```python
from build123d import *

# Parameters (mm, degrees)
BOSS_EXTRUDE1_DEPTH = 1.524
SKETCH2_R           = 7.874
BOSS_EXTRUDE2_DEPTH = 1.524
BOSS_EXTRUDE3_DEPTH = 1.524
CUT_EXTRUDE1_DEPTH  = 1.524


with BuildPart() as part:
    # Sketch1 → Boss-Extrude1 (new body)
    with BuildSketch(Plane(origin=(0, 0, 0), x_dir=(1, 0, 0), z_dir=(0, 1, 0))):
        with BuildLine():
            Line((0, 0), (-38.1, 0))
            Line((-38.1, 0), (-38.1, -12.7))
            ThreePointArc((-38.1, -12.7), (-34.380256121, -21.680256121), (-25.4, -25.4))
            Line((-25.4, -25.4), (0, -25.4))
            Line((0, -25.4), (0, -18.034))
            Line((0, -18.034), (-25.4, -18.034))
            ThreePointArc((-25.4, -18.034), (-30.734, -12.7), (-25.4, -7.366))
            Line((-25.4, -7.366), (0, -7.366))
            Line((0, -7.366), (0, 0))
        make_face()
    extrude(amount=BOSS_EXTRUDE1_DEPTH)

    # Sketch2 → Boss-Extrude2 (add)
    with BuildSketch(Plane.XY):
        with BuildLine():
            Line((0, 0), (0, 29.972))
            Line((0, 29.972), (-22.352, 29.972))
            ThreePointArc((-22.352, 29.972), (-33.48751759, 25.35951759), (-38.1, 14.224))
            Line((-38.1, 14.224), (-38.1, 0))
            Line((-38.1, 0), (0, 0))
        make_face()
        with Locations((-22.352, 14.224)):
            Circle(SKETCH2_R, mode=Mode.SUBTRACT)
    extrude(amount=-BOSS_EXTRUDE2_DEPTH)

    # Sketch3 → Boss-Extrude3 (add)
    with BuildSketch(Plane(origin=(0, 0, 0), x_dir=(0, 1, 0), z_dir=(0.529919264233206, 0, 0.8480480961564253))):
        with BuildLine():
            Line((29.972, 0), (29.972, -47.498))
            ThreePointArc((29.972, -47.498), (26.330994661, -57.001809762), (17.272, -61.640121482))
            Line((17.272, -61.640121482), (17.272, -54.44479552))
            ThreePointArc((17.272, -54.44479552), (21.289625754, -51.955681909), (22.86, -47.498))
            Line((22.86, -47.498), (22.86, -15.748))
            ThreePointArc((22.86, -15.748), (15.748, -8.636), (8.636, -15.748))
            Line((8.636, -15.748), (8.636, -47.498))
            ThreePointArc((8.636, -47.498), (10.206374246, -51.955681909), (14.224, -54.44479552))
            Line((14.224, -54.44479552), (14.224, -61.640121482))
            ThreePointArc((14.224, -61.640121482), (5.165005339, -57.001809762), (1.524, -47.498))
            Line((1.524, -47.498), (1.524, 0))
            Line((1.524, 0), (29.972, 0))
        make_face()
    extrude(amount=-BOSS_EXTRUDE3_DEPTH)

    # Sketch4 → Cut-Extrude1 (cut)
    with BuildSketch(Plane.XZ):
        Polygon((0, 0), (-0.436999968, -1.524), (0, -1.524), align=None)
    extrude(amount=-CUT_EXTRUDE1_DEPTH, mode=Mode.SUBTRACT)


solid = part.part
```
Source: CAD feature listing. Evaluate the final solid. Frame: model axes, mm. A direction names the side the tool comes from. Coordinates: 2 decimals unless noted, no trailing zeros. Write each loop counter-clockwise with the first axis right and the second up, starting at its lowest first coordinate (ties: lowest second). Pieces come first, ordered by that corner, then holes. Notation, with made-up numbers: M -0.75,15.25 L 50.25,15.25 A22 ccw 50.25,43.25 Z; hole C -30,-39.5 d4. An arc over 180 degrees is marked long. Answer as a JSON object with one key per item and string values.
1. Access query for faces 1 (the flat face through (-19, 1.524, 7)), 2 (the cylindrical face through (43.618, 10.164, -28.142)), 3 (the flat face through (-15, 19, -1.524)). Directions: +Z, -Z, +X, -X, +Y, -Y. A direction counts if a zero-diameter tool reaches every point of the face in a straight line with its end or side. Return the directions, or none.
Evaluation:
{"face 1": "+Z, +X, -X, +Y", "face 2": "+Z, -X", "face 3": "-Z, -X, +Y, -Y"}
2. Draft query along X for faces 4 (the flat face through (9, 29.972, -7)), 5 (the cylindrical face through (-14.84, 16.59, -0.75)), 6 (the cylindrical face through (-34.48, 0.75, 21.58)). Return one class per face: released by +X, released by -X, zero draft, split by the parting line, or undercut.
Evaluation:
{"face 4": "zero draft", "face 5": "undercut", "face 6": "released by -X"}
3. Contact query for flat-ended pins moving along their axis: P1, Ø1.5, axis at x = 48.5, z = -30.5, coming from the -Y side; P2, Ø1.5, axis at x = -7.5, y = 24.5, coming from the -Z side; P3, Ø1.2, axis at y = 1, z = 20.5, coming from the +X side. Output: stop coordinate, or through.
Evaluation:
{"P1": "y = 4.77", "P2": "z = -1.52", "P3": "x = 0"}
4. Cut plane B-B on z = -22.5. Output: boundary loops of the cut face in (x, y), plus the area to 3 significant figures.
Evaluation:
{"outline": "M 33.13,1.52 L 36.01,1.52 L 36.01,8.64 L 33.13,8.64 Z; M 33.13,22.86 L 36.01,22.86 L 36.01,29.97 L 33.13,29.97 Z", "area": "40.9 mm^2"}
5. Cut plane A-A on x = -8.5. Output: boundary loops of the cut face in (y, z), plus the area to 3 significant figures.
Evaluation:
{"outline": "M 0,-1.52 L 29.97,-1.52 L 29.97,0 L 1.52,0 L 1.52,7.37 L 0,7.37 Z; M 0,18.03 L 1.52,18.03 L 1.52,25.4 L 0,25.4 Z", "area": "68.1 mm^2"}
6. Cut plane C-C on y = 15.5. Output: boundary loops of the cut face in (x, z).
Evaluation:
{"outline": "M -38.05,-1.52 L -30.12,-1.52 L -30.12,0 L -38.05,0 Z; M -14.58,-1.52 L -0.44,-1.52 L 6.52,-5.87 L 7.33,-4.58 L 0,0 L -14.58,0 Z"}
7. Cut plane D-D on y = 25. Output: boundary loops of the cut face in (x, z).
Evaluation:
{"outline": "M -33.84,-1.52 L -0.44,-1.52 L 48.64,-32.19 L 49.44,-30.9 L 0,0 L -33.84,0 Z"}
8. Ray query, L1, parallel to Z at x = -3.5, y = 20.25; L2, parallel to Y at x = -0.5, z = 21.5; L3, parallel to Z at x = 0, y = 18.25. Return the intervals inside material, ascending.
Evaluation:
{"L1": "-1.52 to 0", "L2": "0 to 1.52", "L3": "-1.8 to 0"}
